```python
from build123d import *

# Parameters (mm, degrees)
SKETCH1_W                           = 28
SKETCH1_H                           = 15
BOSS_EXTRUDE1_DEPTH                 = 4
SKETCH2_W                           = 2
SKETCH2_H                           = 14
BOSS_EXTRUDE2_DEPTH                 = 2
SKETCH3_W                           = 2
SKETCH3_H                           = 11
BOSS_EXTRUDE3_DEPTH                 = 7.5
FILLET1_R                           = 10
CUT_EXTRUDE5_REACH                  = 33.313
CUT_EXTRUDE5_END_RADIUS             = 10
CUT_EXTRUDE5_DIRECTION_2_REACH      = 33.313
CUT_EXTRUDE5_DIRECTION_2_END_RADIUS = 10
BOSS_EXTRUDE4_DEPTH                 = 5
CUT_EXTRUDE6_DEPTH                  = 2
CUT_EXTRUDE6_DEPTH_BACK             = 15
SKETCH22_W                          = 21
SKETCH22_H                          = 5.222778623
BOSS_EXTRUDE6_START                 = -1.5
BOSS_EXTRUDE6_DEPTH                 = 1.75
CUT_EXTRUDE7_REACH                  = 43.938
SKETCH25_W                          = 4.745430675
SKETCH25_H                          = 15
CUT_EXTRUDE7_DIRECTION_2_REACH      = 43.938
SKETCH26_R                          = 1.55
CUT_EXTRUDE8_DEPTH                  = 4
SKETCH27_R                          = 3
CUT_EXTRUDE9_DEPTH                  = 2.5


with BuildPart() as part:
    # Sketch1 → Boss-Extrude1 (new body)
    with BuildSketch(Plane(origin=(0, 0, 0), x_dir=(1, 0, 0), z_dir=(0, 1, 0))):
        Rectangle(SKETCH1_W, SKETCH1_H)
    extrude(amount=BOSS_EXTRUDE1_DEPTH)

    # Sketch2 → Boss-Extrude2 (add, symmetric)
    with BuildSketch(Plane.XY):
        with Locations((-11.5, 11)):
            Rectangle(SKETCH2_W, SKETCH2_H)
        Polygon((-8.5, 15), (-10.5, 18), (-10.5, 15), align=None)
        Polygon((8.5, 15), (10.5, 15), (10.5, 18), align=None)
        with Locations((11.5, 11)):
            Rectangle(SKETCH2_W, SKETCH2_H)
    extrude(amount=BOSS_EXTRUDE2_DEPTH, both=True)

    # Sketch3 → Boss-Extrude3 (add, symmetric)
    with BuildSketch(Plane.XY):
        with Locations((-11.5, 9.5)):
            Rectangle(SKETCH3_W, SKETCH3_H)
        with Locations((11.5, 9.5)):
            Rectangle(SKETCH3_W, SKETCH3_H)
    extrude(amount=BOSS_EXTRUDE3_DEPTH, both=True)

    # Fillet1
    # the kernel refuses this fillet: 10 mm, written as the material it adds along each edge
    with BuildSketch(Plane(origin=(12.5, 4, -7.5), x_dir=(1, 0, 0), z_dir=(0, 0, 1))) as fillet1_piece_1:
        with BuildLine():
            CenterArc((10, 5.267826876), FILLET1_R, 180, 31.788330617)
            Line((0, 5.267826876), (-0.2, 5.267826876))
            Line((-0.2, 5.267826876), (-0.2, 0))
            Line((-0.2, 0), (0, -0.2))
            ThreePointArc((0, -0.2), (0.75, -0.2), (1.33, -0.105356538))
            Line((1.33, -0.105356538), (1.5, 0))
        make_face()
    extrude(amount=15)
    with BuildSketch(Plane(origin=(-12.5, 4, 7.5), x_dir=(0, 1, 0), z_dir=(0, 0, -1))) as fillet1_piece_2:
        with BuildLine():
            CenterArc((5.267826876, -10), FILLET1_R, 90, 31.788330617)
            Line((0, -1.5), (-0.105356538, -1.33))
            ThreePointArc((-0.105356538, -1.33), (-0.2, -0.75), (-0.2, 0))
            Line((-0.2, 0), (0, 0.2))
            Line((0, 0.2), (5.267826876, 0.2))
            Line((5.267826876, 0.2), (5.267826876, 0))
        make_face()
    extrude(amount=15)

    # Cut-Extrude5: up to this cylinder (the profile starts outside it)
    cut_extrude5_end = Plane(origin=(-22.5, 9.267826876, 5.390493), z_dir=(0, 0, -1)) * Cylinder(CUT_EXTRUDE5_END_RADIUS, 87.626, mode=Mode.PRIVATE)
    # Sketch13 → Cut-Extrude5 (cut, up to the surface)
    with BuildSketch(Plane(origin=(-10.5, 0, 0), x_dir=(0, 0, -1), z_dir=(1, 0, 0)), mode=Mode.PRIVATE) as cut_extrude5_sk1:
        Polygon((-3.5, 15), (-6, 15), (-7.5, 15), (-7.5, 8.718379218), (-6, 8.718379218), (-6, 7), (-3.5, 7), align=None)
    cut_extrude5_tool1 = extrude(cut_extrude5_sk1.sketch, amount=-CUT_EXTRUDE5_REACH, mode=Mode.PRIVATE) - cut_extrude5_end
    add(cut_extrude5_tool1.solids().sort_by_distance((-10.5, 11.275152, 5.390493))[0], mode=Mode.SUBTRACT)

    # Cut-Extrude5 direction 2: up to this cylinder (the profile starts outside it)
    cut_extrude5_direction_2_end = Plane(origin=(22.5, 9.267826876, 5.390493), z_dir=(0, 0, 1)) * Cylinder(CUT_EXTRUDE5_DIRECTION_2_END_RADIUS, 87.626, mode=Mode.PRIVATE)
    # Sketch13 → Cut-Extrude5 direction 2 (cut, up to the surface)
    with BuildSketch(Plane(origin=(-10.5, 0, 0), x_dir=(0, 0, -1), z_dir=(1, 0, 0)), mode=Mode.PRIVATE) as cut_extrude5_direction_2_sk1:
        Polygon((-3.5, 15), (-6, 15), (-7.5, 15), (-7.5, 8.718379218), (-6, 8.718379218), (-6, 7), (-3.5, 7), align=None)
    cut_extrude5_direction_2_tool1 = extrude(cut_extrude5_direction_2_sk1.sketch, amount=CUT_EXTRUDE5_DIRECTION_2_REACH, mode=Mode.PRIVATE) - cut_extrude5_direction_2_end
    add(cut_extrude5_direction_2_tool1.solids().sort_by_distance((-10.5, 11.275152, 5.390493))[0], mode=Mode.SUBTRACT)

    # Sketch14 → Boss-Extrude4 (add)
    with BuildSketch(Plane(origin=(-10.5, 0, 0), x_dir=(0, 0, -1), z_dir=(1, 0, 0))):
        with BuildLine():
            Line((-3.5, 9.727178029), (-3.5, 7))
            Line((-3.5, 7), (-6, 7))
            Line((-6, 7), (-6, 9.727178029))
            ThreePointArc((-6, 9.727178029), (-4.75, 4), (-3.5, 9.727178029))
        make_face()
    boss_extrude4 = extrude(amount=-BOSS_EXTRUDE4_DEPTH)

    # Sweep3: sweep along a path in Sketch17
    with BuildLine(Plane.XY.offset(5)) as sweep3_path:
        Line((-22.411313552, 14), (-11.517237777, 3.105924225))
    # Sketch21 → Sweep3 (sweep)
    with BuildSketch(Plane(origin=(-18.205656776, 18.205656776, 0), x_dir=(-0.7071067811865509, -0.7071067811865441, 0), z_dir=(0.7071067811865441, -0.7071067811865509, 0))):
        with BuildLine():
            Line((6.01040764, -6), (6.01040764, -3.5))
            Line((6.01040764, -3.5), (3.283229611, -3.5))
            ThreePointArc((3.283229611, -3.5), (9.01040764, -4.75), (3.283229611, -6))
            Line((3.283229611, -6), (6.01040764, -6))
        make_face()
    sweep3 = sweep(path=sweep3_path.line)

    # Mirror1: Boss-Extrude4, Sweep3 across plane
    add(boss_extrude4.mirror(Plane(origin=(0, 0, 0), x_dir=(0, 0, 1), z_dir=(1, 0, 0))))
    add(sweep3.mirror(Plane(origin=(0, 0, 0), x_dir=(0, 0, 1), z_dir=(1, 0, 0))))

    # Sketch22 → Cut-Extrude6 (cut, two sides: drawn at the far end of the back side and taken through both)
    with BuildSketch(Plane.XY.offset(7.5).offset(-CUT_EXTRUDE6_DEPTH_BACK)):
        with Locations((0, 6.611389311)):
            Rectangle(SKETCH22_W, SKETCH22_H)
    extrude(amount=CUT_EXTRUDE6_DEPTH + CUT_EXTRUDE6_DEPTH_BACK, mode=Mode.SUBTRACT)

    # Sketch24 → Boss-Extrude6 (add)
    with BuildSketch(Plane.XY.offset(7.5).offset(BOSS_EXTRUDE6_START)):
        Polygon((-10.5, 9.727178029), (-12.5, 9.727178029), (-12.5, 3.956694639), (-14, 3.956694639), (-14, 0), (14, 0), (14, 4.212052915), (12.5, 4.212052915), (12.5, 9.727178029), (10.5, 9.727178029), (10.5, 4), (-10.5, 4), align=None)
    extrude(amount=BOSS_EXTRUDE6_DEPTH)

    # Cut-Extrude7: up to this face of the body (flat: up to its plane)
    cut_extrude7_end = Plane(part.part.faces().sort_by_distance((14, 1.807333916, -0.907267183))[0])
    # Sketch25 → Cut-Extrude7 (cut, up to the picked face)
    with BuildSketch(Plane.ZY.offset(12.5), mode=Mode.PRIVATE) as cut_extrude7_sk1:
        with Locations((-5.127284663, 7.5)):
            Rectangle(SKETCH25_W, SKETCH25_H)
    cut_extrude7_tool1 = split(extrude(cut_extrude7_sk1.sketch, amount=-CUT_EXTRUDE7_REACH, mode=Mode.PRIVATE), bisect_by=cut_extrude7_end, keep=Keep.BOTH, mode=Mode.PRIVATE)
    add(cut_extrude7_tool1.solids().sort_by(Axis((-12.5, 7.5, -5.127285), (1, 0, 0)))[0], mode=Mode.SUBTRACT)

    # Cut-Extrude7 direction 2: up to this face of the body (flat: up to its plane)
    cut_extrude7_direction_2_end = Plane(part.part.faces().sort_by_distance((-14, 1.805327472, -0.914845046))[0])
    # Sketch25 → Cut-Extrude7 direction 2 (cut, up to the picked face)
    with BuildSketch(Plane.ZY.offset(12.5), mode=Mode.PRIVATE) as cut_extrude7_direction_2_sk1:
        with Locations((-5.127284663, 7.5)):
            Rectangle(SKETCH25_W, SKETCH25_H)
    cut_extrude7_direction_2_tool1 = split(extrude(cut_extrude7_direction_2_sk1.sketch, amount=CUT_EXTRUDE7_DIRECTION_2_REACH, mode=Mode.PRIVATE), bisect_by=cut_extrude7_direction_2_end, keep=Keep.BOTH, mode=Mode.PRIVATE)
    add(cut_extrude7_direction_2_tool1.solids().sort_by(Axis((-12.5, 7.5, -5.127285), (-1, 0, 0)))[0], mode=Mode.SUBTRACT)

    # Sketch26 → Cut-Extrude8 (cut)
    with BuildSketch(Plane(origin=(0, 4, 0), x_dir=(1, 0, 0), z_dir=(0, 1, 0))):
        with Locations(Location((0, -2.495430675, 0), (0, 0, 270))):
            Circle(SKETCH26_R)
    extrude(amount=-CUT_EXTRUDE8_DEPTH, mode=Mode.SUBTRACT)

    # Sketch27 → Cut-Extrude9 (cut)
    with BuildSketch(Plane(origin=(0, 4, 0), x_dir=(1, 0, 0), z_dir=(0, 1, 0))):
        with Locations(Location((0, -2.495430675, 0), (0, 0, 270))):
            Circle(SKETCH27_R)
    extrude(amount=-CUT_EXTRUDE9_DEPTH, mode=Mode.SUBTRACT)


solid = part.part
```
Read the model definition and answer for the solid it produces. Units are mm, in the model's axes. A direction names the side the tool comes from. Round coordinates to 2 decimals unless told otherwise and drop trailing zeros. Write each loop counter-clockwise with the first axis right and the second up, starting at its lowest first coordinate (ties: lowest second). Pieces come first, ordered by that corner, then holes. Notation, with made-up numbers: (-38, 45) - (2, 45) arc R13 ccw to (2, 49) - close; hole circle Ø10 at (61, -5.5). An arc over 180 degrees is marked (long way). One line per item, written item: value.
Q1. Find section A-A (x = 0). Determine the outline of the cut face in (y, z), and give its area (3 significant figures).
The answers:
outline: (0, -2.75) - (4, -2.75) - (4, -0.5) - (1.5, -0.5) - (1.5, 0.95) - (0, 0.95) - close; (0, 4.05) - (1.5, 4.05) - (1.5, 5.5) - (4, 5.5) - (4, 7.75) - (0, 7.75) - close
area: 22.4 mm2
Q2. Straight lines are drawn through the part: line 1 (X direction, y = 9.25, z = 0); line 2 (Y direction, x = 1, z = 6.75); line 3 (Y direction, x = -2, z = 1.25). For each, find the intervals that lie inside material, in ascending order. Write a range as from..to.
The answers:
line 1: x = -12.5..-10.5, 10.5..12.5
line 2: y = 0..4
line 3: y = 0..1.5
Q3. Which of the six approach directions +Z, -Z, +X, -X, +Y, -Y give full straight-line access (tool end or side, diameter ignored) to faces 5 (the flat face through (18.9, 10.4, 4.7)), 6 (the flat face through (11, 17, -2)), 7 (the flat face through (-11, 9.727, 7))?
The answers:
face 5: +Y
face 6: -Z, +X, -X, +Y
face 7: +Z, +Y
Q4. Find section C-C (z = 6.5). Determine the outline of the cut face in (x, y).
The answers:
outline: (-24.18, 12.23) - (-14, 2.05) - (-14, 0) - (14, 0) - (14, 2.05) - (24.18, 12.23) - (20.73, 15.68) - (14.49, 9.44) - (12.5, 9.44) - (12.5, 9.73) - (10.5, 9.73) - (10.5, 4) - (-10.5, 4) - (-10.5, 9.73) - (-12.5, 9.73) - (-12.5, 9.44) - (-14.49, 9.44) - (-20.73, 15.68) - close
Q5. Find section B-B (z = -1.5). Determine the outline of the cut face in (x, y), and give its area (3 significant figures).
The answers:
outline: (-14, 0) - (14, 0) - (14, 4) arc R10 cw to (12.5, 9.27) - (12.5, 18) - (10.5, 18) - (8.5, 15) - (10.5, 15) - (10.5, 4) - (-10.5, 4) - (-10.5, 15) - (-8.5, 15) - (-10.5, 18) - (-12.5, 18) - (-12.5, 9.27) arc R10 cw to (-14, 4) - close
area: 179 mm2
Q6. For a pull along Y with two mould halves and no side action, classify faces 1 (the flat face through (-16, 11, 6)), 2 (the flat face through (11, 18, 0)), 3 (the flat face through (-10.5, 8, 1)), 4 (the flat face through (9, 15, 0)) as pulls with the +Y half, pulls with the -Y half, needs draft (parallel to the pull), parting line crosses it, or undercut.
The answers:
face 1: needs draft
face 2: pulls with the +Y half
face 3: undercut
face 4: undercut
Q7. Each of these flat-tipped pins is pushed along its axis until it touches: P1, Ø0.8, axis at x = 12, z = 2.5, coming from the +Y side; P2, Ø3, axis at y = 12.5, z = 1, coming from the +X side; P3, Ø0.9, axis at y = 8.5, z = 6.5, coming from the -X side. Where does it stop, or does it pass through?
The answers:
P1: stops at y = 15
P2: stops at x = 23.86
P3: stops at x = -21.05
